Source: CAD feature listing. Evaluate the final solid. Frame: model axes, mm. A direction names the side the tool comes from. Coordinates: 2 decimals unless noted, no trailing zeros. Write each loop counter-clockwise with the first axis right and the second up, starting at its lowest first coordinate (ties: lowest second). Pieces come first, ordered by that corner, then holes. Notation, with made-up numbers: M 7.25,41 L 20.25,41 A27 cw 20.25,68 Z; hole C 74,29.5 d2. An arc over 180 degrees is marked long. Write item = value, one per line. Start each with the question number.
1. Section query B-B (x = 0). Output: boundary loops of the cut face in (y, z).
2. Section query C-C (y = 32.5). Output: boundary loops of the cut face in (x, z), then the cut area to 3 significant figures.
3. Access query for faces 1 (the face through (1, 40, -1)), 2 (the face through (45, 20, -23)). Directions: +Z, -Z, +X, -X, +Y, -Y. A direction counts if a zero-diameter tool reaches every point of the face in a straight line with its end or side. Return the directions, or none.
4. Section query A-A (z = 0). Output: boundary loops of the cut face in (x, y), then the cut area to 3 significant figures.
5. Pin query (flat end, axial travel): pin 1 Ø10 at (x, z) = (32.5, -60) entering from -Y; pin 2 Ø1 at (x, y) = (27, 35) entering from +Z; pin 3 Ø12 at (y, z) = (9, 28) entering from +X. Return the tip coordinate at first contact, or that it passes through.
6. Line query: line 1 along Y through (x, z) = (-57.5, 5.5); line 2 along Z through (x, y) = (-57.5, 29); line 3 along X through (y, z) = (30.5, -33). Output: solid intervals per line, ascending.
```python
from build123d import *

# Parameters (mm, degrees)
SKETCH1_R           = 50
BOSS_EXTRUDE1_DEPTH = 20
SKETCH2_R           = 75
BOSS_EXTRUDE2_DEPTH = 20
FILLET1_R           = 15
FILLET3_R           = 10


with BuildPart() as part:
    # Sketch1 → Boss-Extrude1 (new body)
    with BuildSketch(Plane(origin=(0, 0, 0), x_dir=(1, 0, 0), z_dir=(0, 1, 0))):
        with Locations(Location((0, 0, 0), (0, 0, 270))):
            Circle(SKETCH1_R)
    extrude(amount=BOSS_EXTRUDE1_DEPTH)

    # Sketch2 → Boss-Extrude2 (add)
    with BuildSketch(Plane(origin=(0, 20, 0), x_dir=(1, 0, 0), z_dir=(0, 1, 0))):
        with Locations(Location((0, 0, 0), (0, 0, 270))):
            Circle(SKETCH2_R)
    extrude(amount=BOSS_EXTRUDE2_DEPTH)

    # Fillet1
    fillet1_edges = [part.edges().sort_by_distance(p)[0] for p in [
        (0, 20, -75),
    ]]
    fillet(fillet1_edges, radius=FILLET1_R)

    # Fillet3
    # the kernel refuses this fillet: 10 mm, written as the material it takes off along each edge
    with BuildSketch(Plane(origin=(0, 40, 0), x_dir=(0, 0, 1), z_dir=(-1, 0, 0))) as fillet3_piece_1:
        with BuildLine():
            CenterArc((66.339745962, -10), FILLET3_R, 30, 60)
            Line((66.339745962, 0), (75, 0))
            Line((75, 0), (75, -5))
        make_face()
    revolve(axis=Axis((0, 40, 0), (0, 1, 0)), mode=Mode.SUBTRACT)


solid = part.part
```
Results are:
q1.outline = M 0,-50 L 20,-50 L 20,-60 A15 ccw 35,-75 A10 ccw 40,-66.34 L 40,66.34 A10 ccw 35,75 A15 ccw 20,60 L 20,50 L 0,50 Z
q2.outline = C 0,0 d149.58
q2.area = 17,600 mm^2
q3.face_1 = +Z, -Z, +X, -X, +Y
q3.face_2 = -Y
q4.outline = M -75,35 A15 ccw -60,20 L -50,20 L -50,0 L 50,0 L 50,20 L 60,20 A15 ccw 75,35 A10 ccw 66.34,40 L -66.34,40 A10 ccw Z
q4.area = 4,880 mm^2
q5.pin_1 = 20.35
q5.pin_2 = 70.16
q5.pin_3 = 44.9
q6.line_1 = 20 to 40
q6.line_2 = -46.18 to 46.18
q6.line_3 = -66.58 to 66.58
